Verification items for the finished model (mm, model axes). A direction names the side the tool comes from. Round coordinates to 2 decimals unless told otherwise and drop trailing zeros. Write each loop counter-clockwise with the first axis right and the second up, starting at its lowest first coordinate (ties: lowest second). Pieces come first, ordered by that corner, then holes. Notation, with made-up numbers: M 81.5,59 L 120.5,59 A26 cw 120.5,92 Z; hole C 80,85.25 d11. An arc over 180 degrees is marked long. Write each question's results on one line, items separated by ' | '.
from build123d import *

# Parameters (mm, degrees)
F2_R = 2.54
F3_R = 0.635
F4_R = 0.635


with BuildPart() as f1:
    # F0 (on Front) → F1 (revolve)
    with BuildSketch(Plane.XZ):
        Polygon((-9.756139, 0), (0, 0), (0, 1.523547), (-8.266838, 1.523547), (-8.266838, 28.479891), (-1.564985, 31.905282), (-1.564985, 36.075324), (-2.905356, 36.224253), (-2.905356, 32.947794), (-9.756139, 29.820262), align=None)
    revolve(axis=Axis((0, 0, 0.761774), (0, 0, 1)))

    # F2
    f2_edges = [f1.edges().sort_by_distance(p)[0] for p in [
        (9.756139, 0, 29.820262),
        (9.756139, 0, 0),
        (-9.756139, 0, 14.910131),
    ]]
    fillet(f2_edges, radius=F2_R)

    # F3
    f3_edges = [f1.edges().sort_by_distance(p)[0] for p in [
        (2.905356, 0, 36.224253),
    ]]
    fillet(f3_edges, radius=F3_R)

    # F4
    f4_edges = [f1.edges().sort_by_distance(p)[0] for p in [
        (2.905356, 0, 32.947794),
    ]]
    fillet(f4_edges, radius=F4_R)


solid = f1.part
1) Draft check along Z on faces 4 (the flat face through (0, 0, 0)), 5 (the cylindrical face through (0.339, 1.528, 34.019)), 6 (the conical face through (-1.8, -0.57, 31.74)). Enter one of: pulls with the +Z half, pulls with the -Z half, needs draft (parallel to the pull), parting line crosses it, or undercut.
Calculated:
face 4: pulls with the -Z half | face 5: needs draft | face 6: undercut
2) Access from +Z, -Z, +X, -X, +Y, -Y to the whole of each face (thin tool, end or side, straight path). Record for faces 1 (the cylindrical face through (-2.684, 1.113, 34.42)), 2 (the flat face through (0, 0, 1.524)), 3 (the cylindrical face through (-9.01, 3.74, 15.18)).
Calculated:
face 1: +Z | face 2: none | face 3: +Z, -Z
3) Depth check by flat-ended pin: P1, Ø1, axis at y = 4, z = 14.5, coming from the +X side; P2, Ø1.9, axis at x = 0, y = 0, coming from the +Z side; P3, Ø2, axis at x = 6, z = 27, coming from the -Y side. Enter the tip coordinate at first touch or a pass-through.
Calculated:
P1: stops at x = 9.11 | P2: stops at z = 1.52 | P3: stops at y = -8.38
4) Material ranges on line 1 (X direction, y = 0, z = 10); line 2 (Y direction, x = 0, z = 33.5), recorded low to high. Write a range as [from, to].
Calculated:
line 1: x = [-9.76, -8.27], [8.27, 9.76] | line 2: y = [-2.91, -1.56], [1.56, 2.91]
5) Sectioned sample at A-A, the plane z = 18.5. Record the cut outline in (x, y).
Calculated:
outline: C 0,0 d19.51; hole C 0,0 d16.53
